The model under review builds one solid part; all positions refer to its coordinate system, in mm. A direction names the side the tool comes from. Give positions to 0.01 mm unless a question says otherwise; leave off trailing zeros. Loops run counter-clockwise (first coordinate to the right, second up) from the corner with the lowest first, then second, coordinate; pieces in that order, holes last. Notation, with made-up numbers: M 20,14.5 L 59,14.5 A22 ccw 59,23.5 Z; hole C 56,-4 d9. An arc over 180 degrees is marked long. Put each result on its own line as item: value. Start each with the question number.
Autodesk Fusion 360 part; units mm, degrees
sketch "Skizze1" plane through (0, 0, 0) normal (0, 1, 0) x (1, 0, 0)
  line L0 (0, 0) -> (3, 0)
  line L1 (3, 0) -> (3, 3)
  line L2 (0, 0) -> (0, 3)
  line L3 (3, 3) -> (6.5, 3)
  line L4 (6.5, 3) -> (6.5, 3.4599)
  line L5 (0, 3) -> (-3.5, 3)
  line L6 (1.5, 0) -> (1.5, 47)
  line L7 (1.5, 47) -> (3, 47)
  line L8 (3, 47) -> (0, 47)
  line L9 (0, 47) -> (0, 44)
  line L10 (3, 47) -> (3, 44)
  line L11 (6.5, 3) -> (6.5, 44)
  line L12 (6.5, 44) -> (3, 44)
  line L13 (-3.5, 3) -> (-3.5, 44)
  line L14 (-3.5, 44) -> (0, 44)
  dimension "d1" = 3
  dimension "d2" = 3
  dimension "d3" = 3
  dimension "d4" = 3.5
  dimension "d5" = 3.5
  dimension "d6" = 47
  dimension "d7" = 1.5
  dimension "d8" = 3
  dimension "d9" = 3
extrude "Extrusion1" add sketch "Skizze1" along normal blind 3
Item 1: Consider section B-B, the plane x = -1.75. Write out the cut boundary in (y, z).
Item 2: Consider section A-A, the plane y = 1.85. Write out the cut boundary in (x, z), plus the area to 3 significant figures.
Item 3: To check wall thickness, follow L1, parallel to Z at x = 5, y = 2.05; L2, parallel to X at y = 0.65, z = -2.5. State the ranges of each line that lie inside material, in increasing order. Write a range as [from, to].
Item 4: Clearance check with flat-ended pins moving along their axes: pin 1 Ø0.9 at (y, z) = (2, -1.5) entering from +X; pin 2 Ø1.5 at (x, y) = (4.5, 1) entering from -Z; pin 3 Ø1.5 at (x, y) = (5.5, 1) entering from +Z; pin 4 Ø6 at (x, z) = (4.5, -32) entering from -Y. State where each tip first meets the part, or that it passes through.
Item 5: Tool access review of faces 1 (the flat face through (0, 1, -1)), 2 (the flat face through (5, 1, -44)), 3 (the flat face through (1, 1, 0)), 4 (the flat face through (-2, 1, -44)), 5 (the flat face through (3, 1, -1)): name each direction out of +Z, -Z, +X, -X, +Y, -Y from which nothing blocks a thin tool from reaching the whole face with its end or side.
Report:
1. outline: M 0,-44 L 3,-44 L 3,-3 L 0,-3 Z
2. outline: M -3.5,-44 L 0,-44 L 0,-47 L 3,-47 L 3,-44 L 6.5,-44 L 6.5,-3 L 3,-3 L 3,0 L 0,0 L 0,-3 L -3.5,-3 Z
2. area: 428 mm²
3. L1: [-44, -3]
3. L2: [0, 3]
4. pin 1: x = 3
4. pin 2: z = -44
4. pin 3: z = -3
4. pin 4: y = 0
5. face 1: +Z, -X, +Y, -Y
5. face 2: -Z, +X, +Y, -Y
5. face 3: +Z, +X, -X, +Y, -Y
5. face 4: -Z, -X, +Y, -Y
5. face 5: +Z, +X, +Y, -Y
